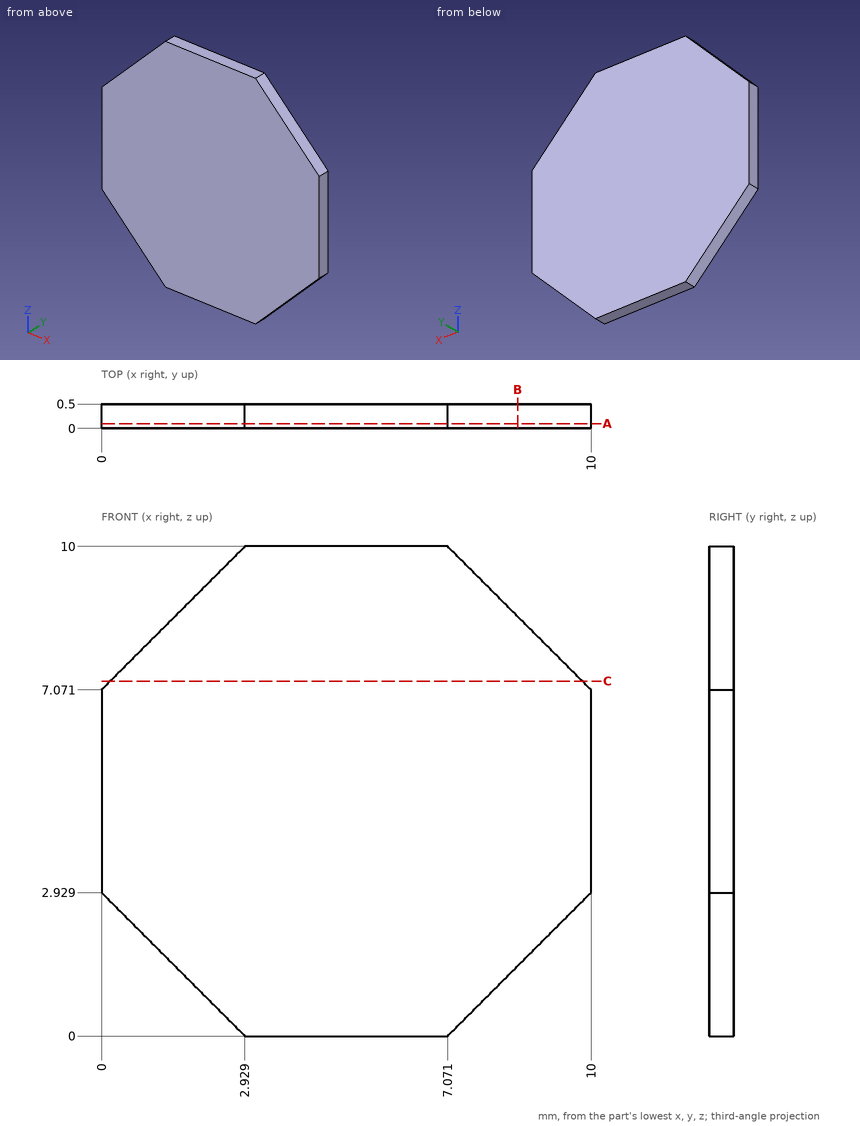
Verification items for this drawing (mm, ordinates from the low corner). Round coordinates to 2 decimals unless told otherwise and drop trailing zeros. Write each loop counter-clockwise with the first axis right and the second up, starting at its lowest first coordinate (ties: lowest second). Pieces come first, ordered by that corner, then holes. Notation, with made-up numbers: (53, 42) - (61, 42) arc R20 ccw to (61, 78) - close; hole circle Ø6 at (-4.5, 83). An arc over 180 degrees is marked (long way). One line per item, written item: value.
1. Cross-section at B-B on x = 8.5. Record the boundary of the cut face in (y, z).
The answers:
outline: (0, 1.43) - (0.5, 1.43) - (0.5, 8.57) - (0, 8.57) - close
2. Cross-section at A-A on y = 0.1. Record the boundary of the cut face in (x, z), and give its area (3 significant figures).
The answers:
outline: (0, 2.93) - (2.93, 0) - (7.07, 0) - (10, 2.93) - (10, 7.07) - (7.07, 10) - (2.93, 10) - (0, 7.07) - close
area: 82.8 mm^2
3. Cross-section at C-C on z = 7.25. Record the boundary of the cut face in (x, y).
The answers:
outline: (0.18, 0) - (9.82, 0) - (9.82, 0.5) - (0.18, 0.5) - close
4. Scan lines: L1, parallel to X at y = 0.2, z = 8.5; L2, parallel to X at y = 0.1, z = 9.75; L3, parallel to Z at x = 8, y = 0.2. Record each from-to range of solid material in increasing order.
The answers:
L1: x = 1.43 to 8.57
L2: x = 2.68 to 7.32
L3: z = 0.93 to 9.07
